Check sheet for the modelled part. Datum: model origin and axes. Units: mm. A direction names the side the tool comes from. Round coordinates to 2 decimals unless told otherwise and drop trailing zeros. Loops run counter-clockwise (first coordinate to the right, second up) from the corner with the lowest first, then second, coordinate; pieces in that order, holes last. Notation, with made-up numbers: M -12.5,-2.5 L 38.5,-2.5 A30 cw 38.5,34.5 Z; hole C -36,40.25 d4. An arc over 180 degrees is marked long. One line per question, with ' | ' between items. Start each with the question number.
(1) Section check D-D (z = -1.75). Record the boundary of the cut face in (x, y).
(2) Tool access check on faces 4 (the face through (-0.325, 3.536, -4.484)), 5 (the face through (2.307, 4.888, 4.436)). Record the directions out of +Z, -Z, +X, -X, +Y, -Y that give a thin tool (end or side, any length) a straight path to the whole face; none if there is none.
(3) Draft check along Y on faces 1 (the face through (-8.6, 21.9, 3)), 2 (the face through (-4, 0, 2)), 3 (the face through (-0.325, 3.536, 4.484)). Enter one of: +Y half, -Y half, draft (parallel to the pull), parting line (faces both ways), or undercut.
(4) Section check B-B (y = 2). Record the boundary of the cut face in (x, z), and give its area (3 significant figures).
(5) Go/stop test with flat-tipped pins: P1, Ø4, axis at x = -3, z = 1.5, coming from the -Y side; P2, Ø3, axis at x = -0.5, z = -1.5, coming from the -Y side; P3, Ø3, axis at y = 14.5, z = 1, coming from the -X side; P4, Ø1.5, axis at x = 0, y = 17, coming from the +Z side. Record where each tip stops, or that it passes through.
(6) Section check A-A (z = 2.75). Record the boundary of the cut face in (x, y), and give its area (3 significant figures).
(7) Section check C-C (x = -0.5). Count the separate pieces of the cut face and the enclosed holes in it, and give its area (3 significant figures).
(8) Thickness scan on probe 1 along Z at (x, y) = (0, 2.5). Record the ranges inside material, lowest first. Write a range as [from, to].
```python
from build123d import *

# Parameters (mm, degrees)
F1_R          = 5
F1_R_2        = 4.25
F3_R          = 1.5
F4_DEPTH      = 25
F4_DEPTH_BACK = 25


with BuildPart() as f2:
    # F2: sweep along a path in F0
    with BuildLine(Plane.XY) as f2_path:
        Line((0, 0), (0, 9.6410161514))
        ThreePointArc((0, 9.6410161514), (-0.6814834742, 14.8173970534), (-2.6794919243, 19.6410161514))
        Line((-2.6794919243, 19.6410161514), (-7.5, 27.9903810568))
    # F1 (on Front) → F2 (sweep)
    with BuildSketch(Plane.XZ):
        Circle(F1_R)
        Circle(F1_R_2, mode=Mode.SUBTRACT)
    sweep(path=f2_path.line)

    # F3 (on Top) → F4 (cut, two sides)
    with BuildSketch(Plane.XY) as f4_sk:
        with Locations((0, 5)):
            Circle(F3_R)
    extrude(amount=-F4_DEPTH, mode=Mode.SUBTRACT)
    extrude(f4_sk.sketch, amount=F4_DEPTH_BACK, mode=Mode.SUBTRACT)


solid = f2.part
```
The answers:
1) outline: M -11.56,25.65 L -6.74,17.3 A15.32 cw -4.68,9.64 L -4.68,0 L -3.87,0 L -3.87,9.64 A16.13 ccw -6.03,17.7 L -10.85,26.05 Z; M -4.15,29.93 L 0.67,21.58 A23.87 cw 3.87,9.64 L 3.87,0 L 4.68,0 L 4.68,9.64 A24.68 ccw 1.38,21.98 L -3.44,30.33 Z
2) face 4: +Z, -Z | face 5: -Y
3) face 1: parting line | face 2: -Y half | face 3: undercut
4) outline: C 0,0 d10; hole C 0,0 d8.5 | area: 21.8 mm²
5) P1: y = 0 | P2: y = 20.78 | P3: x = -6.35 | P4: z = 4.97
6) outline: M -11.12,25.9 L -6.3,17.55 A15.82 cw -4.18,9.64 L -4.18,0 L -3.24,0 L -3.24,9.64 A16.76 ccw -5.49,18.02 L -10.31,26.37 Z; M -4.69,29.61 L 0.13,21.26 A23.24 cw 3.24,9.64 L 3.24,0 L 4.18,0 L 4.18,9.64 A24.18 ccw 0.94,21.73 L -3.88,30.08 Z | area: 55.7 mm²
7) separate pieces: 3 | enclosed holes: 0 | area: 41.5 mm²
8) probe 1: [-5, -4.25], [4.25, 5]
